Here's how the part is built. I have some questions about the finished solid (model axes, mm). Face numbers are marked on the shaded views. A direction names the side the tool comes from. Give positions to 0.01 mm unless a question says otherwise; leave off trailing zeros. Write each loop counter-clockwise with the first axis right and the second up, starting at its lowest first coordinate (ties: lowest second). Pieces come first, ordered by that corner, then holes. Notation, with made-up numbers: (47, -19) -> (99, -19) arc R23 cw to (99, 1) -> close; hole circle Ø10 at (64, -26.5). An arc over 180 degrees is marked (long way). Use one line per item in the form item = value.
```python
from build123d import *

# Parameters (mm, degrees)
EXTRUDE_1_DEPTH = 50
SKETCH_4_R      = 2
EXTRUDE_2_DEPTH = 10
M4X0_7_1_D      = 3.3
M4X0_7_1_DEPTH  = 10.1
M4X0_7_1_TIP    = 0.991420021


with BuildPart() as part:
    # 草圖1 → 填料-伸長1 (new body)
    with BuildSketch(Plane.XY):
        Polygon((-2.309401077, 4), (-4.618802154, 0), (-2.309401077, -4), (2.309401077, -4), (4.618802154, 0), (2.309401077, 4), align=None)
    extrude(amount=EXTRUDE_1_DEPTH)

    # 草圖4 → 填料-伸長2 (add)
    with BuildSketch(Plane(origin=(0, 0, 0), x_dir=(-1, 0, 0), z_dir=(0, 0, -1))):
        Circle(SKETCH_4_R)
    extrude(amount=EXTRUDE_2_DEPTH)

    # M4x0.7 螺紋孔1
    with Locations(Plane.XY.offset(50)):
        with Locations((0, 0)):
            Hole(M4X0_7_1_D / 2, depth=M4X0_7_1_DEPTH)
            with Locations((0, 0, -(M4X0_7_1_DEPTH + M4X0_7_1_TIP / 2))):  # 118° drill point
                Cone(0, M4X0_7_1_D / 2, M4X0_7_1_TIP, mode=Mode.SUBTRACT)


solid = part.part
```
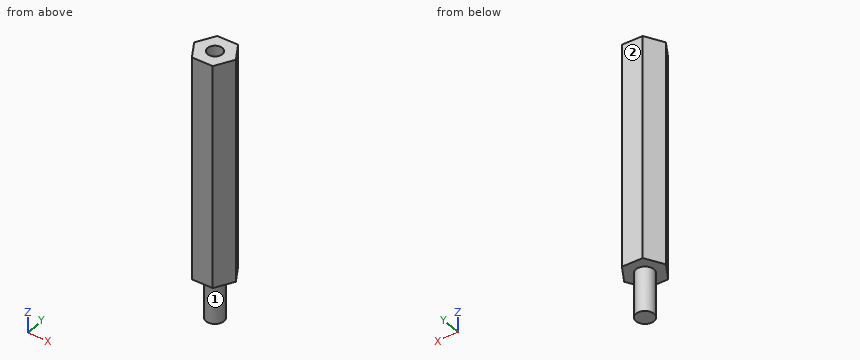
Q1. If I drill on line 1 along X through (y, z) = (0, 46.5); line 2 along Y through (x, z) = (0, 42.5); line 3 along Z through (x, y) = (-0.25, 3.25), over which ranges is the centre line in solid material (lowest first)? Write a range as from..to.
Result set:
line_1 = -4.62..-1.65, 1.65..4.62
line_2 = -4..-1.65, 1.65..4
line_3 = 0..50
Q2. I want a section at A-A, the plane z = 13. Write out the boundary of the cut face in (x, y), and give its area (3 significant figures).
Result set:
outline = (-4.62, 0) -> (-2.31, -4) -> (2.31, -4) -> (4.62, 0) -> (2.31, 4) -> (-2.31, 4) -> close
area = 55.4 mm2
Q3. Which directions (+Z, -Z, +X, -X, +Y, -Y) give clear straight access to the entire face, cutting with the end or side of a thin tool? Please do the marked faces 1 and 2.
Result set:
face_1 = -Z
face_2 = +Z, -Z, +X, -X, +Y
Q4. I want a section at C-C, the plane y = 2.75. Write out the boundary of the cut face in (x, z), and give its area (3 significant figures).
Result set:
outline = (-3.03, 0) -> (3.03, 0) -> (3.03, 50) -> (-3.03, 50) -> close
area = 303 mm2
Q5. Will these pins go through, and if not, where does the flat tip stop? pin 1 Ø1.5 at (y, z) = (-0.5, 21.5) entering from -X; pin 2 Ø3 at (y, z) = (2, 18.5) entering from -X; pin 3 Ø3 at (x, y) = (2.5, -2) entering from -Z; pin 4 Ø1 at (y, z) = (1, 7) entering from +X.
Result set:
pin_1 = -4.62
pin_2 = -4.33
pin_3 = -10
pin_4 = 4.33
Q6. I want a section at B-B, the plane y = -3. Write out the boundary of the cut face in (x, z).
Result set:
outline = (-2.89, 0) -> (2.89, 0) -> (2.89, 50) -> (-2.89, 50) -> close
